Can you work these out from the model? Positions are in its coordinate system, mm. Face numbers are marked on the shaded views. A direction names the side the tool comes from. Give positions to 0.01 mm unless a question says otherwise; leave off trailing zeros. Order: outer loops, then holes, each group sorted by start corner. A loop starts at its lowest first (then second) coordinate and runs counter-clockwise, first axis right, second up. Notation, with made-up numbers: M 72,54.5 L 102,54.5 A24 cw 102,75.5 Z; hole C 29,76 d11. An arc over 180 degrees is marked long. Answer as a JSON object with one key per item and string values.
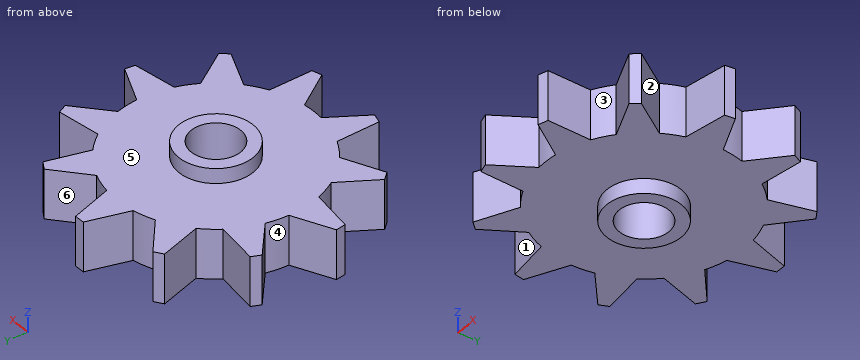
```python
from build123d import *

# Parameters (mm, degrees)
SKETCH1_R                = 20
BOSS_EXTRUDE1_DEPTH      = 10
BOSS_EXTRUDE2_DEPTH      = 3
BOSS_EXTRUDE2_DEPTH_BACK = 13
SKETCH2_R                = 7.5
CUT_EXTRUDE2_DEPTH       = 33.496153619
CUT_EXTRUDE2_DEPTH_BACK  = 33.496153619
SKETCH3_R                = 5
BOSS_EXTRUDE3_DEPTH      = 10


with BuildPart() as part:
    # Sketch1 → Boss-Extrude1 (new body)
    with BuildSketch(Plane.XY):
        Circle(SKETCH1_R)
    extrude(amount=BOSS_EXTRUDE1_DEPTH)

    # Sketch2 → Boss-Extrude2 (add, two sides: drawn at the far end of the back side and taken through both)
    with BuildSketch(Plane.XY.offset(10).offset(-BOSS_EXTRUDE2_DEPTH_BACK)):
        Circle(SKETCH2_R)
    extrude(amount=BOSS_EXTRUDE2_DEPTH + BOSS_EXTRUDE2_DEPTH_BACK)

    # Sketch3 → Cut-Extrude2 (cut, two sides: drawn at the far end of the back side and taken through both)
    with BuildSketch(Plane.XY.offset(13).offset(-CUT_EXTRUDE2_DEPTH_BACK)):
        Circle(SKETCH3_R)
    extrude(amount=CUT_EXTRUDE2_DEPTH + CUT_EXTRUDE2_DEPTH_BACK, mode=Mode.SUBTRACT)

    # Sketch4 → Boss-Extrude3 (add)
    with BuildSketch(Plane.XY.offset(10)):
        Polygon((-1, 28), (1, 28), (4, 18), (-4, 18), align=None)
        Polygon((6.366520583, 17.305126861), (14.296689356, 24.095739737), (15.979196422, 23.014458102), (13.096548846, 12.980000321), align=None)
        Polygon((14.711715864, 11.115998215), (25.054280857, 12.541252359), (25.885110883, 10.721988369), (18.035035968, 3.838942253), align=None)
        Polygon((18.386045307, 1.397618679), (27.857315211, -2.99499403), (27.572685534, -4.974636914), (17.247526601, -6.520952856), align=None)
        Polygon((16.222935274, -8.764494914), (21.815848816, -17.580350976), (20.506127348, -19.091850125), (10.984049403, -14.810491508), align=None)
        Polygon((8.909157918, -16.143943298), (8.848004565, -26.584070704), (6.929018618, -27.147535818), (1.233214129, -18.397803752), align=None)
        Polygon((-1.233214129, -18.397803752), (-6.929018618, -27.147535818), (-8.848004565, -26.584070704), (-8.909157918, -16.143943298), align=None)
        Polygon((-10.984049403, -14.810491508), (-20.506127348, -19.091850125), (-21.815848816, -17.580350976), (-16.222935274, -8.764494914), align=None)
        Polygon((-17.247526601, -6.520952856), (-27.572685534, -4.974636914), (-27.857315211, -2.99499403), (-18.386045307, 1.397618679), align=None)
        Polygon((-18.035035968, 3.838942253), (-25.885110883, 10.721988369), (-25.054280857, 12.541252359), (-14.711715864, 11.115998215), align=None)
        Polygon((-13.096548846, 12.980000321), (-15.979196422, 23.014458102), (-14.296689356, 24.095739737), (-6.366520583, 17.305126861), align=None)
    extrude(amount=-BOSS_EXTRUDE3_DEPTH)


solid = part.part
```
1) I'm going to push flat-ended pins straight in: pin 1 Ø8 at (x, z) = (-21, 0.5) entering from +Y; pin 2 Ø3 at (x, z) = (5, 7.5) entering from -Y; pin 3 Ø4 at (x, y) = (11.5, 8.5) entering from -Z. Where does each tip first touch, or does it pass through?
Results found:
{"pin 1": "stops at y = 12.53", "pin 2": "stops at y = -26.49", "pin 3": "stops at z = 0"}
2) For the marked faces 1, 2 and 3, which set-ups out of +Z, -Z, +X, -X, +Y, -Y let a thin tool reach every point of the face, with its end or its side?
Results found:
{"face 1": "+Z, -Z, -X", "face 2": "+Z, -Z, +X", "face 3": "+Z, -Z, -Y"}
3) Thinking about a two-plate mould opening in Y: for the marked faces 4, 5 and 6, which applies, pulls with the +Y half, pulls with the -Y half, needs draft (parallel to the pull), parting line crosses it, or undercut?
Results found:
{"face 4": "undercut", "face 5": "needs draft", "face 6": "pulls with the +Y half"}
4) I need wall thicknesses on L1, parallel to Y at x = 0, z = 1.5; L2, parallel to X at y = 20, z = 3; L3, parallel to X at y = 22.5, z = 7. Which ranges of each line are inside material? Lowest first, please.
Results found:
{"L1": "y = -20 to -5, 5 to 28", "L2": "x = -15.11 to -9.51, -3.4 to 3.4, 9.51 to 15.11", "L3": "x = -15.83 to -12.43, -2.65 to 2.65, 12.43 to 15.83"}
5) I want a section at B-B on y = 0. Write out the boundary of the cut face in (x, z).
Results found:
{"outline": "M -21.4,0 L -7.5,0 L -7.5,-3 L -5,-3 L -5,13 L -7.5,13 L -7.5,10 L -21.4,10 Z; M 5,-3 L 7.5,-3 L 7.5,0 L 21.4,0 L 21.4,10 L 7.5,10 L 7.5,13 L 5,13 Z"}
6) I want a section at C-C on z = 12. Write out the boundary of the cut face in (x, y).
Results found:
{"outline": "C 0,0 d15; hole C 0,0 d10"}
7) I want a section at A-A on x = 0. Write out the boundary of the cut face in (y, z).
Results found:
{"outline": "M -20,0 L -7.5,0 L -7.5,-3 L -5,-3 L -5,13 L -7.5,13 L -7.5,10 L -20,10 Z; M 5,-3 L 7.5,-3 L 7.5,0 L 28,0 L 28,10 L 7.5,10 L 7.5,13 L 5,13 Z"}
8) I want a section at D-D on x = 22.5. Write out the boundary of the cut face in (y, z).
Results found:
{"outline": "M -5.73,0 L -0.51,0 L -0.51,10 L -5.73,10 Z; M 7.75,0 L 12.19,0 L 12.19,10 L 7.75,10 Z"}
